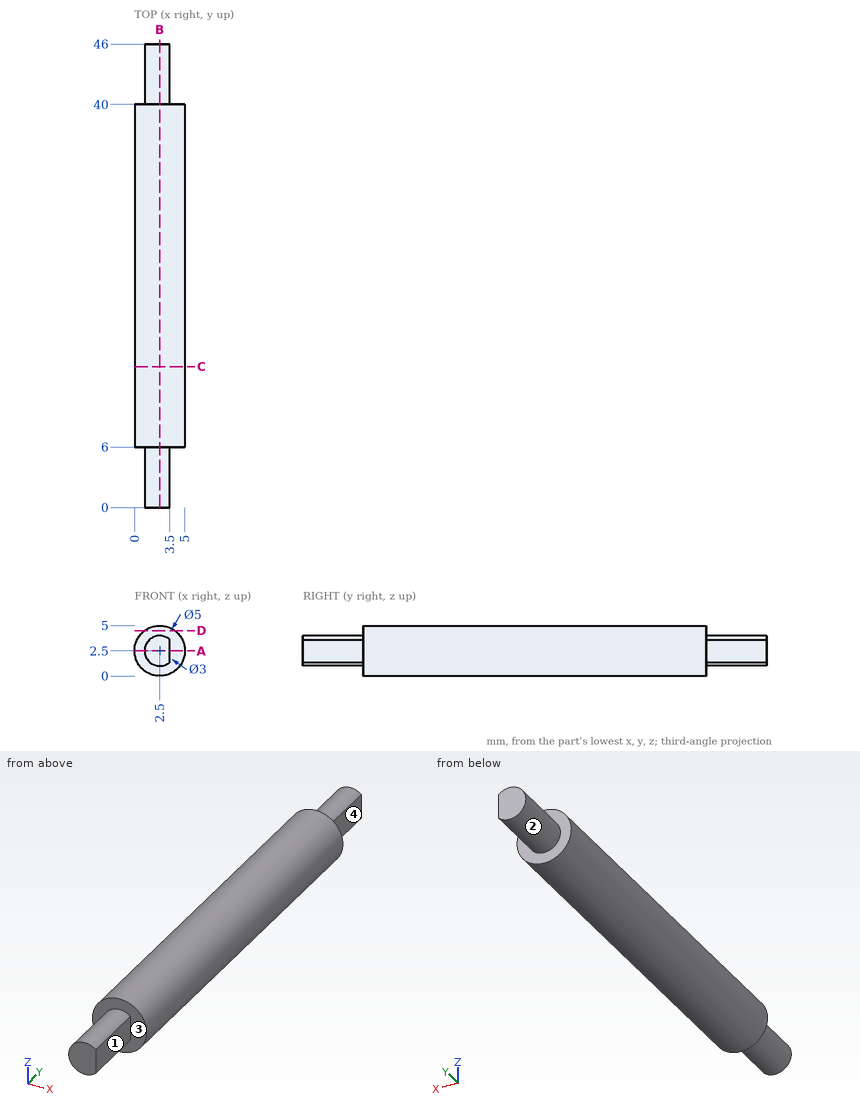
Geometry: see drawing. Coordinates: mm, zero at the bounding-box minimum. A direction names the side the tool comes from. Give positions to 0.01 mm unless a question says otherwise; leave off trailing zeros. Order: outer loops, then holes, each group sorted by start corner. A loop starts at its lowest first (then second) coordinate and runs counter-clockwise, first axis right, second up. Notation, with made-up numbers: (-10.5, 89) -> (27.5, 89) arc R14 ccw to (27.5, 106) -> close; hole circle Ø8 at (33, 55). An arc over 180 degrees is marked (long way). Write each question's results on one line, items separated by ' | '. Start each with the question number.
1) Section A-A (z = 2.5). Return loops of the section in (x, y).
2) Section B-B (x = 2.5). Return loops of the section in (y, z), then the cut area to 3 significant figures.
3) First-contact query: pin 1 (0.7 mm diameter, centred on y = 42.5, z = 2, fed in from +X). Flat tip, straight axial feed; report the tip coordinate or a pass-through.
4) Section C-C (y = 14). Return loops of the section in (x, z).
5) Section D-D (z = 4.5). Return loops of the section in (x, y), then the cut area to 3 significant figures.
6) Set-up query: the marked faces 1, 2, 3 and 4. Return all of +Z, -Z, +X, -X, +Y, -Y with unobstructed straight access to the full face (end or side cutting, diameter ignored); none if empty.
7) Line query: line 1 (Y direction, x = 4.3, z = 3.5); line 2 (X direction, y = 43, z = 2.55); line 3 (Z direction, x = 2.6, y = 3.5). Output: solid intervals per line, ascending. Write a range as from..to.
Calculated:
1) outline: (0, 6) -> (1, 6) -> (1, 0) -> (3.5, 0) -> (3.5, 6) -> (5, 6) -> (5, 40) -> (3.5, 40) -> (3.5, 46) -> (1, 46) -> (1, 40) -> (0, 40) -> close
2) outline: (0, 1) -> (6, 1) -> (6, 0) -> (40, 0) -> (40, 1) -> (46, 1) -> (46, 4) -> (40, 4) -> (40, 5) -> (6, 5) -> (6, 4) -> (0, 4) -> close | area: 206 mm2
3) pin 1: x = 3.5
4) outline: circle Ø5 at (2.5, 2.5)
5) outline: (1, 6) -> (4, 6) -> (4, 40) -> (1, 40) -> close | area: 102 mm2
6) face 1: +Z, -Z, +X, -Y | face 2: +Y | face 3: -Y | face 4: +Z, -Z, +X, +Y
7) line 1: 6..40 | line 2: 1..3.5 | line 3: 1..4
